Build history of the part. All positions in model axes, mm. Face numbers are marked on the shaded views. A direction names the side the tool comes from. Round coordinates to 2 decimals unless told otherwise and drop trailing zeros. Loops run counter-clockwise (first coordinate to the right, second up) from the corner with the lowest first, then second, coordinate; pieces in that order, holes last. Notation, with made-up numbers: M -1,21.5 L 33,21.5 A25 cw 33,51.5 Z; hole C 83.25,83.25 d11. An arc over 180 degrees is marked long. One line per item, written item: value.
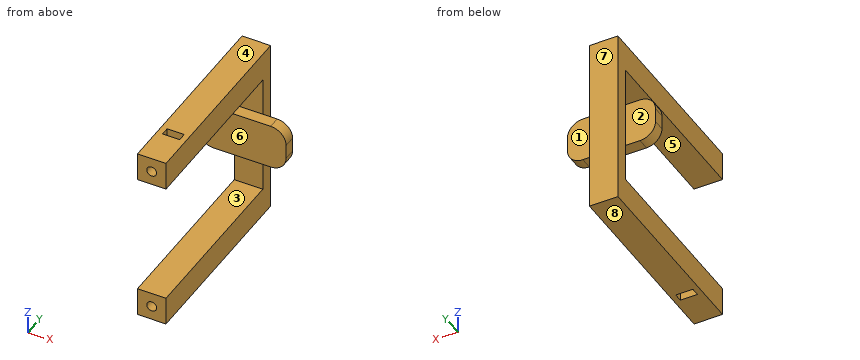
```python
from build123d import *

# Parameters (mm, degrees)
ESQUISSE1_W             = 37
ESQUISSE1_H             = 19
BOSS_EXTRU_1_DEPTH      = 5
CONG_1_R                = 6.5
ESQUISSE4_W             = 12
ESQUISSE4_H             = 75
BOSS_EXTRU_2_DEPTH      = 6
ESQUISSE5_W             = 12
ESQUISSE5_H             = 12
BOSS_EXTRU_3_DEPTH      = 74.7
ESQUISSE6_R             = 2.075
ENL_V_MAT_EXTRU_1_DEPTH = 40
ESQUISSE7_W             = 7.2
ESQUISSE7_H             = 3.5
ENL_V_MAT_EXTRU_2_DEPTH = 10.25
ESQUISSE8_W             = 7.2
ESQUISSE8_H             = 3.5
ENL_V_MAT_EXTRU_3_DEPTH = 10.25


with BuildPart() as part:
    # Esquisse1 → Boss.-Extru.1 (new body)
    with BuildSketch(Plane(origin=(0, 0, 0), x_dir=(1, 0, 0), z_dir=(0, 1, 0))):
        with Locations((-4.867406947, 1.932441033)):
            Rectangle(ESQUISSE1_W, ESQUISSE1_H)
    extrude(amount=BOSS_EXTRU_1_DEPTH)

    # Congé1
    cong_1_edges = [part.edges().sort_by_distance(p)[0] for p in [
        (-23.367406947, 2.5, -11.432441033),
        (13.632593053, 2.5, -11.432441033),
        (13.632593053, 2.5, 7.567558967),
        (-23.367406947, 2.5, 7.567558967),
    ]]
    fillet(cong_1_edges, radius=CONG_1_R)

    # Esquisse4 → Boss.-Extru.2 (add)
    with BuildSketch(Plane(origin=(0, 5, 0), x_dir=(1, 0, 0), z_dir=(0, 1, 0))):
        with Locations((-4.867406947, 1.932441033)):
            Rectangle(ESQUISSE4_W, ESQUISSE4_H)
    extrude(amount=BOSS_EXTRU_2_DEPTH)

    # Esquisse5 → Boss.-Extru.3 (add)
    with BuildSketch(Plane(origin=(0, 5, 0), x_dir=(-1, 0, 0), z_dir=(0, -1, 0))):
        with Locations((4.867406947, 33.432441033)):
            Rectangle(ESQUISSE5_W, ESQUISSE5_H)
        with Locations((4.867406947, -29.567558967)):
            Rectangle(ESQUISSE5_W, ESQUISSE5_H)
    extrude(amount=BOSS_EXTRU_3_DEPTH)

    # Esquisse6 → Enlèv. mat.-Extru.1 (cut)
    with BuildSketch(Plane.XZ.offset(69.7)):
        with Locations(Location((-4.867406947, 29.567558967, 0), (0, 0, 270))):
            Circle(ESQUISSE6_R)
        with Locations(Location((-4.867406947, -33.432441033, 0), (0, 0, 270))):
            Circle(ESQUISSE6_R)
    extrude(amount=-ENL_V_MAT_EXTRU_1_DEPTH, mode=Mode.SUBTRACT)

    # Esquisse7 → Enlèv. mat.-Extru.2 (cut)
    with BuildSketch(Plane.XY.offset(35.567558967)):
        with Locations((-4.867406947, -52.95)):
            Rectangle(ESQUISSE7_W, ESQUISSE7_H)
    extrude(amount=-ENL_V_MAT_EXTRU_2_DEPTH, mode=Mode.SUBTRACT)

    # Esquisse8 → Enlèv. mat.-Extru.3 (cut)
    with BuildSketch(Plane(origin=(0, 0, -39.432441033), x_dir=(-1, 0, 0), z_dir=(0, 0, -1))):
        with Locations((4.867406947, -52.95)):
            Rectangle(ESQUISSE8_W, ESQUISSE8_H)
    extrude(amount=-ENL_V_MAT_EXTRU_3_DEPTH, mode=Mode.SUBTRACT)


solid = part.part
```
Item 1: Slice it at A-A, the plane y = -4. Give the cut face in (x, z).
Check values:
outline: M -10.87,-39.43 L 1.13,-39.43 L 1.13,-27.43 L -10.87,-27.43 Z; M -10.87,23.57 L 1.13,23.57 L 1.13,35.57 L -10.87,35.57 Z
Item 2: Drop flat-ended pins along their axis: P1, Ø6, axis at x = -18, z = 0.5, coming from the +Y side; P2, Ø1, axis at y = -53.5, z = -36.5, coming from the -X side; P3, Ø1.5, axis at x = -18, y = -1, coming from the -Z side; P4, Ø6, axis at x = -4, z = 28, coming from the -Y side. Give the stop position or say it passes through.
Check values:
P1: stops at y = 5
P2: stops at x = -10.87
P3: passes through
P4: stops at y = -69.7
Item 3: Pull direction Z, two halves, no side cores. Call the marked faces 5, 6, 7 and 8: pulls with the +Z half, pulls with the -Z half, needs draft (parallel to the pull), parting line crosses it, or undercut.
Check values:
face 5: undercut
face 6: undercut
face 7: needs draft
face 8: pulls with the -Z half
Item 4: Which spindle directions (+Z, -Z, +X, -X, +Y, -Y) get a long thin tool onto all of the face, cutting with end or side? Do the marked faces 1, 2, 3 and 4. Say none if no direction does.
Check values:
face 1: +Z, -Z, +X, +Y
face 2: +Z, -Z, -X, +Y
face 3: +X, -X, -Y
face 4: +Z, +X, -X, +Y, -Y
Item 5: Slice it at D-D, the plane z = 28.5. Give the cut face in (x, y).
Check values:
outline: M -10.87,-69.7 L -6.65,-69.7 L -6.65,-54.7 L -8.47,-54.7 L -8.47,-51.2 L -6.65,-51.2 L -6.65,-29.7 L -3.09,-29.7 L -3.09,-51.2 L -1.27,-51.2 L -1.27,-54.7 L -3.09,-54.7 L -3.09,-69.7 L 1.13,-69.7 L 1.13,11 L -10.87,11 Z
Item 6: Wall check: line 1 along Y through (x, z) = (-15, -4); line 2 along X through (y, z) = (-33, -30); line 3 along Z through (x, y) = (-3.5, -33.5). Give the ranges that are in metal, low to high.
Check values:
line 1: y = 0 to 5
line 2: x = -10.87 to 1.13
line 3: z = -39.43 to -34.99, -31.87 to -27.43, 23.57 to 28.01, 31.13 to 35.57
Item 7: Slice it at C-C, the plane x = 0. Give the cut face in (y, z), and give its area (3 significant figures).
Check values:
outline: M -69.7,-39.43 L 11,-39.43 L 11,35.57 L -69.7,35.57 L -69.7,23.57 L 5,23.57 L 5,7.57 L 0,7.57 L 0,-11.43 L 5,-11.43 L 5,-27.43 L -69.7,-27.43 Z
area: 2,340 mm2
Item 8: Slice it at B-B, the plane y = -50. Give the cut face in (x, z) (3 decimals).
Check values:
outline: M -10.867,-39.432 L 1.133,-39.432 L 1.133,-27.432 L -10.867,-27.432 Z; M -10.867,23.568 L 1.133,23.568 L 1.133,35.568 L -10.867,35.568 Z; hole C -4.867,-33.432 d4.15; hole C -4.867,29.568 d4.15
